Can you work these out from the model? Positions are in its coordinate system, mm. A direction names the side the tool comes from. Coordinates: 2 decimals unless noted, no trailing zeros.
```python
from build123d import *

# Parameters (mm, degrees)
EXTRUDE_1_DEPTH     = 120
SKETCH_2_R          = 3
CUT_EXTRUDE_1_DEPTH = 4.5
SKETCH_3_R          = 1.75
CUT_EXTRUDE_2_DEPTH = 121.421136019


with BuildPart() as part:
    # 草图1 → 凸台-拉伸1 (new body)
    with BuildSketch(Plane.XY):
        with BuildLine():
            ThreePointArc((6.2, 9), (6.412132034, 8.912132034), (6.5, 8.7))
            Line((6.5, 8.7), (6.5, 0.3))
            ThreePointArc((6.5, 0.3), (6.412132034, 0.087867966), (6.2, 0))
            Line((6.2, 0), (5.557669683, 0))
            ThreePointArc((5.557669683, 0), (5.444280341, 0.035249106), (5.370859728, 0.128571429))
            ThreePointArc((5.370859728, 0.128571429), (5.130846451, 0.514929157), (4.764285714, 0.784209483))
            ThreePointArc((4.764285714, 0.784209483), (4.680969149, 0.858006567), (4.65, 0.964911064))
            Line((4.65, 0.964911064), (4.65, 1))
            ThreePointArc((4.65, 1), (4.25, 1.4), (3.85, 1))
            Line((3.85, 1), (3.85, 0.964911064))
            ThreePointArc((3.85, 0.964911064), (3.819030851, 0.858006567), (3.735714286, 0.784209483))
            ThreePointArc((3.735714286, 0.784209483), (3.369153549, 0.514929157), (3.129140272, 0.128571429))
            ThreePointArc((3.129140272, 0.128571429), (3.055719659, 0.035249106), (2.942330317, 0))
            Line((2.942330317, 0), (0.6, 0))
            Line((0.6, 0), (0, 0.6))
            Line((0, 0.6), (0, 8.4))
            Line((0, 8.4), (0.6, 9))
            Line((0.6, 9), (2.942330317, 9))
            ThreePointArc((2.942330317, 9), (3.055719659, 8.964750894), (3.129140272, 8.871428571))
            ThreePointArc((3.129140272, 8.871428571), (3.369153549, 8.485070843), (3.735714286, 8.215790517))
            ThreePointArc((3.735714286, 8.215790517), (3.819030851, 8.141993433), (3.85, 8.035088936))
            Line((3.85, 8.035088936), (3.85, 8))
            ThreePointArc((3.85, 8), (4.25, 7.6), (4.65, 8))
            Line((4.65, 8), (4.65, 8.035088936))
            ThreePointArc((4.65, 8.035088936), (4.680969149, 8.141993433), (4.764285714, 8.215790517))
            ThreePointArc((4.764285714, 8.215790517), (5.130846451, 8.485070843), (5.370859728, 8.871428571))
            ThreePointArc((5.370859728, 8.871428571), (5.444280341, 8.964750894), (5.557669683, 9))
            Line((5.557669683, 9), (6.2, 9))
        make_face()
    extrude(amount=EXTRUDE_1_DEPTH)

    # 草图2 → 切除-拉伸1 (cut)
    with BuildSketch(Plane(origin=(6.5, 0, 0), x_dir=(0, 0, -1), z_dir=(1, 0, 0))):
        with Locations((-10, 4.5)):
            Circle(SKETCH_2_R)
        with Locations((-30, 4.5)):
            Circle(SKETCH_2_R)
        with Locations((-50, 4.5)):
            Circle(SKETCH_2_R)
        with Locations((-70, 4.5)):
            Circle(SKETCH_2_R)
        with Locations((-90, 4.5)):
            Circle(SKETCH_2_R)
        with Locations((-110, 4.5)):
            Circle(SKETCH_2_R)
        with Locations((-130, 4.5)):
            Circle(SKETCH_2_R)
        with Locations((-150, 4.5)):
            Circle(SKETCH_2_R)
        with Locations((-170, 4.5)):
            Circle(SKETCH_2_R)
        with Locations((-190, 4.5)):
            Circle(SKETCH_2_R)
        with Locations((-210, 4.5)):
            Circle(SKETCH_2_R)
        with Locations((-230, 4.5)):
            Circle(SKETCH_2_R)
        with Locations((-250, 4.5)):
            Circle(SKETCH_2_R)
        with Locations((-270, 4.5)):
            Circle(SKETCH_2_R)
        with Locations((-290, 4.5)):
            Circle(SKETCH_2_R)
        with Locations((-310, 4.5)):
            Circle(SKETCH_2_R)
        with Locations((-330, 4.5)):
            Circle(SKETCH_2_R)
        with Locations((-350, 4.5)):
            Circle(SKETCH_2_R)
        with Locations((-370, 4.5)):
            Circle(SKETCH_2_R)
        with Locations((-390, 4.5)):
            Circle(SKETCH_2_R)
        with Locations((-410, 4.5)):
            Circle(SKETCH_2_R)
        with Locations((-430, 4.5)):
            Circle(SKETCH_2_R)
        with Locations((-450, 4.5)):
            Circle(SKETCH_2_R)
        with Locations((-470, 4.5)):
            Circle(SKETCH_2_R)
        with Locations((-490, 4.5)):
            Circle(SKETCH_2_R)
    extrude(amount=-CUT_EXTRUDE_1_DEPTH, mode=Mode.SUBTRACT)

    # 草图3 → 切除-拉伸2 (cut, through all)
    with BuildSketch(Plane(origin=(2, 0, 0), x_dir=(0, 0, -1), z_dir=(1, 0, 0))):
        with Locations((-10, 4.5)):
            Circle(SKETCH_3_R)
        with Locations((-30, 4.5)):
            Circle(SKETCH_3_R)
        with Locations((-50, 4.5)):
            Circle(SKETCH_3_R)
        with Locations((-70, 4.5)):
            Circle(SKETCH_3_R)
        with Locations((-90, 4.5)):
            Circle(SKETCH_3_R)
        with Locations((-110, 4.5)):
            Circle(SKETCH_3_R)
        with Locations((-130, 4.5)):
            Circle(SKETCH_3_R)
        with Locations((-150, 4.5)):
            Circle(SKETCH_3_R)
        with Locations((-170, 4.5)):
            Circle(SKETCH_3_R)
        with Locations((-190, 4.5)):
            Circle(SKETCH_3_R)
        with Locations((-210, 4.5)):
            Circle(SKETCH_3_R)
        with Locations((-230, 4.5)):
            Circle(SKETCH_3_R)
        with Locations((-250, 4.5)):
            Circle(SKETCH_3_R)
        with Locations((-270, 4.5)):
            Circle(SKETCH_3_R)
        with Locations((-290, 4.5)):
            Circle(SKETCH_3_R)
        with Locations((-310, 4.5)):
            Circle(SKETCH_3_R)
        with Locations((-330, 4.5)):
            Circle(SKETCH_3_R)
        with Locations((-350, 4.5)):
            Circle(SKETCH_3_R)
        with Locations((-370, 4.5)):
            Circle(SKETCH_3_R)
        with Locations((-390, 4.5)):
            Circle(SKETCH_3_R)
        with Locations((-410, 4.5)):
            Circle(SKETCH_3_R)
        with Locations((-430, 4.5)):
            Circle(SKETCH_3_R)
        with Locations((-450, 4.5)):
            Circle(SKETCH_3_R)
        with Locations((-470, 4.5)):
            Circle(SKETCH_3_R)
        with Locations((-490, 4.5)):
            Circle(SKETCH_3_R)
    extrude(amount=-CUT_EXTRUDE_2_DEPTH, mode=Mode.SUBTRACT)


solid = part.part
```
1. Imagine slicing it at A-A on y = 4.5. Give the number of separate pieces and of enclosed holes in the cut face, then the cut area to 3 significant figures.
Completed:
separate pieces: 7
enclosed holes: 0
area: 576 mm2
2. Thinking about a two-plate mould opening in Y: for faces 1 (the flat face through (3, 5, 120)), 2 (the cylindrical face through (4.3, 4.6, 93)), 3 (the flat face through (2, 0, 59)), which applies, pulls with the +Y half, pulls with the -Y half, needs draft (parallel to the pull), parting line crosses it, or undercut?
Completed:
face 1: needs draft
face 2: undercut
face 3: pulls with the -Y half
3. Please list where these lines run through material, in increasing order: probe 1 along Y at (x, z) = (0.45, 10); probe 2 along Y at (x, z) = (1.25, 110); probe 3 along X at (y, z) = (8, 103).
Completed:
probe 1: y = 0.15 to 2.75, 6.25 to 8.85
probe 2: y = 0 to 2.75, 6.25 to 9
probe 3: x = 0 to 3.85, 4.65 to 6.5
4. On a 3-axis mill with a long thin cutter (end or side, diameter ignored), from which of +Z, -Z, +X, -X, +Y, -Y can I reach the whole of each face in a straight line? I mean faces 4 (the flat face through (2, 2.5, 90)), 5 (the cylindrical face through (1.01, 2.95, 9.19)). Say none if no direction works.
Completed:
face 4: +X
face 5: +X, -X
5. I'm going to push a flat-ended pin straight in: pin 1 (4.5 mm diameter, centred on y = 4.5, z = 90, fed in from +X). Where does the tip first touch, or does it pass through?
Completed:
pin 1: stops at x = 2
